Input: dimensioned drawing with shaded views. Units: mm. Origin: part minimum x, y, z. Give positions to 0.01 mm unless a question says otherwise; leave off trailing zeros. Write each loop counter-clockwise with the first axis right and the second up, starting at its lowest first coordinate (ties: lowest second). Pieces come first, ordered by that corner, then holes. Notation, with made-up numbers: (81, -27) -> (131, -27) arc R21 cw to (131, -4) -> close; hole circle Ø2 at (21.25, 11). An arc over 180 degrees is marked (long way). Answer as a JSON object with one key per item and string values. Group by question number.
(1) Section query C-C on y = 0.35. Output: boundary loops of the cut face in (x, z), plus the area to 3 significant figures.
(2) Section query D-D on x = 27.5. Output: boundary loops of the cut face in (y, z).
(3) Section query A-A on x = 14.5. Output: boundary loops of the cut face in (y, z), plus the area to 3 significant figures.
(4) Section query B-B on z = 6.5. Output: boundary loops of the cut face in (x, y), plus the area to 3 significant figures.
(5) Contact query for a flat-ended pin moving along its axis: pin 1 Ø0.8 at (x, y) = (28, 0.5) entering from +Z. Output: stop coordinate, or through.
(6) Material intervals for probe 1 along Z at (x, y) = (12, 1.05); probe 2 along Z at (x, y) = (26.5, 1.1); probe 3 along Z at (x, y) = (23, 0.3), sorted ascending.
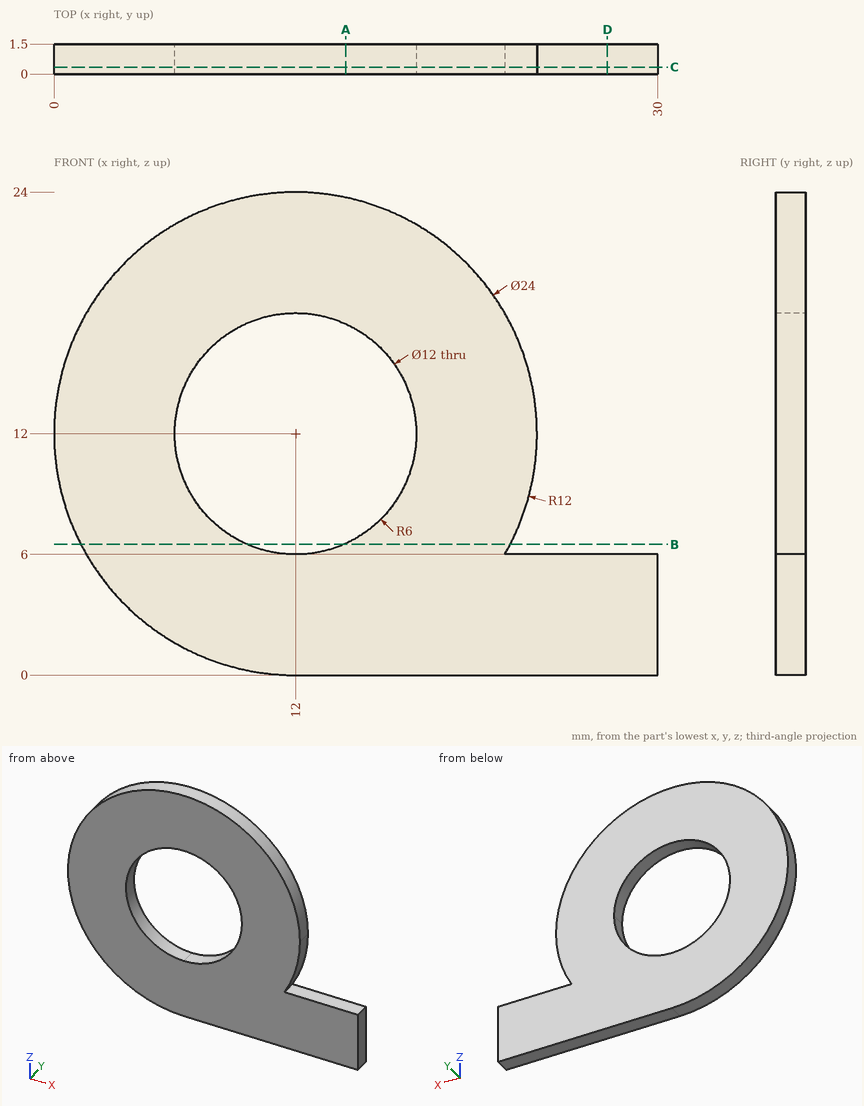
Answer list:
{
 "1": {"outline": "(12, 0) -> (30, 0) -> (30, 6) -> (22.39, 6) arc R12 ccw to (24, 12) arc R12 ccw (long way) to start; hole (12, 6) arc R6 ccw to (18, 12) arc R6 ccw (long way) to start", "area": "403 mm2"},
 "2": {"outline": "(0, 0) -> (1.5, 0) -> (1.5, 6) -> (0, 6) -> close"},
 "3": {"outline": "(0, 0) -> (1.5, 0) -> (1.5, 6.55) -> (0, 6.55) -> close; (0, 17.45) -> (1.5, 17.45) -> (1.5, 23.74) -> (0, 23.74) -> close", "area": "19.2 mm2"},
 "4": {"outline": "(1.33, 0) -> (9.6, 0) -> (9.6, 1.5) -> (1.33, 1.5) -> close; (14.4, 0) -> (22.67, 0) -> (22.67, 1.5) -> (14.4, 1.5) -> close", "area": "24.8 mm2"},
 "5": {"pin 1": "z = 6"},
 "6": {"probe 1": "0 to 6, 18 to 24", "probe 2": "0 to 6", "probe 3": "0 to 6, 7.2 to 16.8"}
}
